```python
from build123d import *


with BuildPart() as part:
    # Sketch1 → Revolve1 (revolve)
    with BuildSketch(Plane(origin=(0, 0, 0), x_dir=(0, 0, -1), z_dir=(1, 0, 0))):
        with BuildLine():
            Line((-1.445971311, 4.65), (-1.445971311, 5.15))
            Line((-1.445971311, 5.15), (-1.845971311, 5.15))
            Line((-1.845971311, 5.15), (-3.076316722, 5.1))
            Line((-3.076316722, 5.1), (-3.376316722, 5.1))
            Line((-3.376316722, 5.1), (-3.376316722, 4.65))
            ThreePointArc((-3.376316722, 4.65), (-3.094232719, 2.332601245), (-3, 0))
            Line((-3, 0), (0, 0))
            add(Edge.make_bspline(
                [(0, 0), (-2.675e-06, 0.01666667), (-8.026e-06, 0.050000025), (-8.7895e-05, 0.100000022), (-0.000180393, 0.150000063), (-0.000330536, 0.200000094), (-0.000537467, 0.250000053), (-0.000759597, 0.300000137), (-0.001044147, 0.350000117), (-0.001363821, 0.400000131), (-0.001720577, 0.450000201), (-0.00213388, 0.500000168), (-0.00258391, 0.550000181), (-0.003070489, 0.60000027), (-0.003614151, 0.650000216), (-0.004192925, 0.700000245), (-0.004814168, 0.750000245), (-0.005470422, 0.80000036), (-0.006184171, 0.850000281), (-0.006932922, 0.900000314), (-0.007724172, 0.95000031), (-0.008550424, 1.000000449), (-0.009434173, 1.050000346), (-0.010352924, 1.100000384), (-0.011314174, 1.150000375), (-0.012310428, 1.200000538), (-0.013364176, 1.250000411), (-0.014452926, 1.300000453), (-0.015584178, 1.35000044), (-0.016750427, 1.400000627), (-0.017974197, 1.450000475), (-0.019232861, 1.500000524), (-0.020534438, 1.550000498), (-0.021869472, 1.600000744), (-0.023267779, 1.650000343), (-0.024679493, 1.700000784), (-0.026154367, 1.750000567), (-0.027663148, 1.800000617), (-0.029213151, 1.850000635), (-0.030804364, 1.900000609), (-0.03242952, 1.9500009), (-0.034117709, 2.000000417), (-0.035819762, 2.050000932), (-0.037583409, 2.100000712), (-0.039386752, 2.150000479), (-0.041209716, 2.200000999), (-0.043094579, 2.250000713), (-0.045012147, 2.300000823), (-0.046977008, 2.350000513), (-0.048959975, 2.400001074), (-0.051003318, 2.450000827), (-0.053086955, 2.500000545), (-0.055189036, 2.55000118), (-0.057357151, 2.60000056), (-0.059542551, 2.650000917), (-0.061772874, 2.700000922), (-0.064046189, 2.750000631), (-0.06634257, 2.800000963), (-0.068683782, 2.850000923), (-0.071062569, 2.900000997), (-0.073486209, 2.950000672), (-0.075932824, 3.000001012), (-0.078422781, 3.050001033), (-0.080956347, 3.100000695), (-0.083512081, 3.150001096), (-0.086115631, 3.200000753), (-0.088745651, 3.250000758), (-0.091402026, 3.300001143), (-0.09410657, 3.350000729), (-0.096831979, 3.400001174), (-0.099605857, 3.450000789), (-0.102404883, 3.500000851), (-0.105234896, 3.55000086), (-0.108095823, 3.600000814), (-0.110982119, 3.650001235), (-0.113916085, 3.70000082), (-0.116873864, 3.750000961), (-0.119868764, 3.800000474), (-0.122871331, 3.850001333), (-0.125926314, 3.90000084), (-0.129003762, 3.950001006), (-0.132118968, 4.00000048), (-0.135240638, 4.05000143), (-0.1384189, 4.100000495), (-0.141604042, 4.150001022), (-0.144825285, 4.200000953), (-0.148075192, 4.250000967), (-0.151354329, 4.300001033), (-0.154667867, 4.350000584), (-0.157994497, 4.400001036), (-0.16135453, 4.450001045), (-0.164747775, 4.500000605), (-0.168111531, 4.549367846), (-0.170360364, 4.582067388), (-0.17146867, 4.598100522)],
                knots=[0, 0, 0, 0, 0.010742815, 0.02148564, 0.032228476, 0.042971338, 0.053714238, 0.064457166, 0.075200149, 0.085943183, 0.096686276, 0.107429451, 0.118172701, 0.128916031, 0.139659472, 0.150403009, 0.161146649, 0.171890399, 0.182634296, 0.193378319, 0.204122474, 0.214866768, 0.225611246, 0.236355879, 0.247100673, 0.257845636, 0.268590819, 0.279336185, 0.290081743, 0.300827498, 0.311573509, 0.322319734, 0.333066179, 0.34381285, 0.354559815, 0.365306961, 0.376054417, 0.386802129, 0.397550104, 0.408298349, 0.41904687, 0.429795747, 0.440544842, 0.451294309, 0.462044083, 0.47279409, 0.483544495, 0.494295227, 0.505046292, 0.515797611, 0.526549363, 0.537301469, 0.548053845, 0.558806679, 0.569559793, 0.580313286, 0.591067166, 0.60182134, 0.612575913, 0.62333089, 0.63408628, 0.644841984, 0.655598111, 0.666354669, 0.677111555, 0.687868884, 0.698626549, 0.709384555, 0.720143021, 0.730901836, 0.741661123, 0.752420769, 0.763180777, 0.773941152, 0.784701896, 0.79546314, 0.806224762, 0.816986768, 0.827749031, 0.838511813, 0.84927499, 0.860038566, 0.870802409, 0.881566792, 0.892331448, 0.903096516, 0.913862001, 0.924627905, 0.935394234, 0.946160847, 0.95692789, 0.967695368, 0.978463137, 0.988822257, 0.988822257, 0.988822257, 0.988822257], degree=3))
            Line((-0.17146867, 4.598100522), (-0.42146867, 4.598100522))
            Line((-0.42146867, 4.598100522), (-0.945971311, 4.65))
            Line((-0.945971311, 4.65), (-1.445971311, 4.65))
        make_face()
    revolve(axis=Axis((0, 0, -5.189127774), (0, 0, 1)))


solid = part.part
```
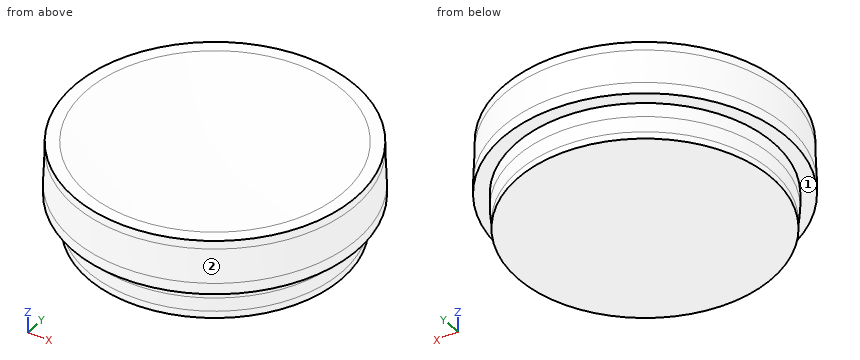
Input: part model. Units: mm. Frame: model coordinates. Face numbers are marked on the shaded views. Coordinates: 2 decimals unless noted, no trailing zeros. Loops run counter-clockwise (first coordinate to the right, second up) from the corner with the lowest first, then second, coordinate; pieces in that order, holes last. Notation, with made-up numbers: (70, 78) -> (107, 78) arc R30 cw to (107, 117) -> close; hole circle Ø1 at (3, -39.75). An arc over 180 degrees is marked (long way). Use a Markdown table: item, result.
1) Cut plane A-A (z = 2.85). Return the cut outline in (x, y).
Results found:
| item | result |
|---|---|
| outline | circle Ø10.22 at (0, 0) |
2) Cut plane B-B (z = 0.8). Return the cut outline in (x, y).
Results found:
| item | result |
|---|---|
| outline | circle Ø9.27 at (0, 0) |
3) Material intervals for line 1 along Z through (x, y) = (4.25, -2.25); line 2 along Y through (x, z) = (0, 1.35); line 3 along Y through (x, z) = (3.25, 0.7), sorted ascending. Write a range as from..to.
Results found:
| item | result |
|---|---|
| line 1 | z = 1.45..3.38 |
| line 2 | y = -4.65..4.65 |
| line 3 | y = -3.29..3.29 |
4) Contact query for flat-ended pins moving along their axis: pin 1 (2 mm diameter, centred on x = 3, y = 1, fed in from -Z); pin 2 (1.5 mm diameter, centred on y = -2, z = 2, fed in from -X); pin 3 (1.5 mm diameter, centred on x = -3, y = 1.5, fed in from -Z). Output: stop coordinate, or through.
Results found:
| item | result |
|---|---|
| pin 1 | stops at z = 0.04 |
| pin 2 | stops at x = -4.99 |
| pin 3 | stops at z = 0.06 |
5) Pull-direction query (Y, two-part tool) for the marked faces 1 and 2; classes: released by +Y, released by -Y, zero draft, split by the parting line, or undercut.
Results found:
| item | result |
|---|---|
| face 1 | zero draft |
| face 2 | split by the parting line |
